Source: CAD feature listing. Evaluate the final solid. Frame: model axes, mm. A direction names the side the tool comes from. Round coordinates to 2 decimals unless told otherwise and drop trailing zeros. Write each loop counter-clockwise with the first axis right and the second up, starting at its lowest first coordinate (ties: lowest second). Pieces come first, ordered by that corner, then holes.
Autodesk Inventor part; units mm, degrees
ref_plane "Work Plane2" through (-89, -40.3889, 33.5) normal (0, 0, 1) x (1, 0, 0)
ref_plane "YZ Plane" through (0, 0, 0) normal (1, 0, 0) x (0, 1, 0)
ref_plane "XZ Plane" through (0, 0, 0) normal (0, 1, 0) x (-1, 0, 0)
ref_plane "Work Plane1" through (0, 0, 0) normal (0, 0, 1) x (1, 0, 0)
sketch "Sketch1" plane through (0, 0, 0) normal (0, 0, 1) x (1, 0, 0)
  line L0 (23.5, 88.5) -> (-23.5, 88.5)
  line L1 (-23.5, 88.5) -> (-23.5, 36.5)
  line L2 (-26.5, 33.5) -> (-89, 33.5)
  line L3 (-89, 33.5) -> (-89, -72.5)
  line L4 (-89, -72.5) -> (-77, -72.5)
  line L5 (-74, -75.5) -> (-74, -93.5)
  line L6 (-74, -93.5) -> (74, -93.5)
  line L7 (74, -93.5) -> (74, -75.5)
  line L8 (77, -72.5) -> (89, -72.5)
  line L9 (89, -72.5) -> (89, 33.5)
  line L10 (89, 33.5) -> (26.5, 33.5)
  line L11 (23.5, 36.5) -> (23.5, 88.5)
  line L12 (-4.5, 81.5) -> (-4.5, 36.5)
  line L13 (-7.5, 33.5) -> (-13.5, 33.5)
  line L14 (-16.5, 36.5) -> (-16.5, 81.5)
  line L15 (-13.5, 84.5) -> (-7.5, 84.5)
  line L16 (16.5, 81.5) -> (16.5, 36.5)
  line L17 (13.5, 33.5) -> (7.5, 33.5)
  line L18 (4.5, 36.5) -> (4.5, 81.5)
  line L19 (7.5, 84.5) -> (13.5, 84.5)
  line L20 (16.5, 88.5) -> (22.5, 88.5)
  line L21 (22.5, 88.5) -> (22.5, 3.75)
  line L22 (22.5, 3.75) -> (16.5, 3.75)
  line L23 (16.5, 3.75) -> (16.5, 88.5)
  line L24 (59.9, 4.75) -> (32.2, 4.75)
  arc A0 (13.5, 33.5) -> (16.5, 36.5) centre (13.5, 36.5) ccw
  arc A1 (4.5, 36.5) -> (7.5, 33.5) centre (7.5, 36.5) ccw
  arc A2 (7.5, 84.5) -> (4.5, 81.5) centre (7.5, 81.5) ccw
  arc A3 (16.5, 81.5) -> (13.5, 84.5) centre (13.5, 81.5) ccw
  arc A4 (-4.5, 81.5) -> (-7.5, 84.5) centre (-7.5, 81.5) ccw
  arc A5 (-7.5, 33.5) -> (-4.5, 36.5) centre (-7.5, 36.5) ccw
  arc A6 (-16.5, 36.5) -> (-13.5, 33.5) centre (-13.5, 36.5) ccw
  arc A7 (-13.5, 84.5) -> (-16.5, 81.5) centre (-13.5, 81.5) ccw
  arc A8 (-26.5, 33.5) -> (-23.5, 36.5) centre (-26.5, 36.5) ccw
  arc A9 (-74, -75.5) -> (-77, -72.5) centre (-77, -75.5) ccw
  arc A10 (77, -72.5) -> (74, -75.5) centre (77, -75.5) ccw
  arc A11 (23.5, 36.5) -> (26.5, 33.5) centre (26.5, 36.5) ccw
  point P0 (0, 0)
  dimension "d0" = 1
  dimension "d1" = 1
ref_plane "Work Plane2" through (-89, -40.3889, 33.5) normal (0, 0, 1) x (1, 0, 0)
extrude "Extrusion1" add sketch "Sketch1" along normal up to surface (33.5 mm away) contours L21 L22 L23 L16 L0
sketch "Sketch2" plane through (22.5, 3.75, 0) normal (1, 0, 0) x (0, 0, -1)
  circle A0 centre (-15.375, 14.375) radius 6.75
  circle A1 centre (-10.5, 57.25) radius 5.5
  point P0 (0, -3.75)
  dimension "d8" = 11
extrude "Extrusion2" cut sketch "Sketch2" against normal up to next
sketch "Sketch3" plane through (16.5, 3.75, 0) normal (-1, 0, 0) x (0, 0, 1)
  circle A0 centre (21.2694, 29.2497) radius 2
  point P0 (0, -3.75)
extrude "Extrusion3" cut sketch "Sketch3" against normal blind 5
properties part number "left_gear_holder"
1) Pull-direction query (Z, two-part tool) for faces 3 (the face through (19, 47, 0)), 4 (the face through (18.96, 34.69, 22.34)), 5 (the face through (20, 88.5, 17)); classes: released by +Z, released by -Z, zero draft, split by the parting line, or undercut.
Taken from the geometry:
face 3: released by -Z
face 4: undercut
face 5: zero draft
2) Section query A-A on y = 61. Return the cut outline in (x, z), then the cut area to 3 significant figures.
Taken from the geometry:
outline: (16.5, 0) - (22.5, 0) - (22.5, 5) - (16.5, 5) - close; (16.5, 16) - (22.5, 16) - (22.5, 33.5) - (16.5, 33.5) - close
area: 135 mm2
3) Contact query for flat-ended pins moving along their axis: P1, Ø12, axis at y = 18.125, z = 15.375, coming from the +X side; P2, Ø1.2, axis at y = 33.5, z = 21, coming from the -X side. Output: stop coordinate, or through.
Taken from the geometry:
P1: passes through
P2: stops at x = 21.5
4) Section query C-C on x = 19.15. Return the cut outline in (y, z) (3 decimals), then the cut area to 3 significant figures.
Taken from the geometry:
outline: (3.75, 0) - (88.5, 0) - (88.5, 33.5) - (3.75, 33.5) - close; hole circle Ø13.5 at (18.125, 15.375); hole circle Ø4 at (33, 21.269); hole circle Ø11 at (61, 10.5)
area: 2,590 mm2
5) Reachability of faces 1 (the face through (21.5, 33, 21)), 2 (the face through (22.5, 47, 17)) from +Z, -Z, +X, -X, +Y, -Y: full face, straight path, thin tool, end or side. Return the list, or none.
Taken from the geometry:
face 1: -X
face 2: +Z, -Z, +X, +Y, -Y
6) Section query D-D on y = 13. Return the cut outline in (x, z).
Taken from the geometry:
outline: (16.5, 0) - (22.5, 0) - (22.5, 10.98) - (16.5, 10.98) - close; (16.5, 19.77) - (22.5, 19.77) - (22.5, 33.5) - (16.5, 33.5) - close
7) Section query B-B on z = 10.5. Return the cut outline in (x, y).
Taken from the geometry:
outline: (16.5, 3.75) - (22.5, 3.75) - (22.5, 13.46) - (16.5, 13.46) - close; (16.5, 22.79) - (22.5, 22.79) - (22.5, 55.5) - (16.5, 55.5) - close; (16.5, 66.5) - (22.5, 66.5) - (22.5, 88.5) - (16.5, 88.5) - close
8) Material intervals for line 1 (Y direction, x = 21.5, z = 11); line 2 (Y direction, x = 20.9, z = 19.5); line 3 (Y direction, x = 19.05, z = 5.5), sorted ascending.
Taken from the geometry:
line 1: y = 3.75 to 12.98, 23.27 to 55.52, 66.48 to 88.5
line 2: y = 3.75 to 12.78, 23.47 to 32.07, 33.93 to 88.5
line 3: y = 3.75 to 58.71, 63.29 to 88.5
